```python
from build123d import *

# Parameters (mm, degrees)
F0_W      = 254
F0_H      = 409.575
F1_DEPTH  = 184.15
F2_W      = 193.675
F2_H      = 476.25
F3_DEPTH  = 95.25
F5_R      = 30.1625
F6_DEPTH  = 25.4
F7_R      = 26.9875
F8_DEPTH  = 25.4
F9_R      = 82.55
F10_DEPTH = 19.05
F11_W     = 177.8
F11_H     = 15.875
F12_DEPTH = 136.525
F14_DEPTH = 60.325
F16_DEPTH = 193.675
F17_R     = 9.525
F18_DEPTH = 38.1
F19_W     = 19.05
F19_H     = 63.5
F20_DEPTH = 12.7


with BuildPart() as f1:
    # F0 (on Top) → F1 (new body)
    with BuildSketch(Plane.XY):
        Rectangle(F0_W, F0_H)
    extrude(amount=F1_DEPTH)

    # F2 (on face) → F3 (join)
    with BuildSketch(Plane.XY.offset(184.15)):
        with Locations((30.1625, -33.3375)):
            Rectangle(F2_W, F2_H)
    extrude(amount=F3_DEPTH)

    # F5 (on face) → F6 (join)
    with BuildSketch(Plane.YZ.offset(127)):
        with Locations((141.2875, 90.4875)):
            Circle(F5_R)
    extrude(amount=F6_DEPTH)

    # F7 (on face) → F8 (cut)
    with BuildSketch(Plane.YZ.offset(152.4)):
        with Locations((141.2875, 90.4875)):
            Circle(F7_R)
    extrude(amount=-F8_DEPTH, mode=Mode.SUBTRACT)

    # F9 (on face) → F10 (join)
    with BuildSketch(Plane(origin=(-127, 0, 0), x_dir=(0, -1, 0), z_dir=(-1, 0, 0))):
        with Locations((-134.9375, 247.65)):
            Circle(F9_R)
    extrude(amount=F10_DEPTH)

    # F11 (on face) → F12 (join)
    with BuildSketch(Plane(origin=(-146.05, 0, 0), x_dir=(0, -1, 0), z_dir=(-1, 0, 0))):
        with Locations((-134.9375, 233.3625)):
            Rectangle(F11_W, F11_H)
    extrude(amount=F12_DEPTH)

    # F13 (on face) → F14 (join, through all)
    with BuildSketch(Plane(origin=(-66.675, 0, 0), x_dir=(0, -1, 0), z_dir=(-1, 0, 0))):
        with BuildLine():
            Line((-204.7875, 279.4), (-204.7875, 184.15))
            Line((-204.7875, 184.15), (15.268247, 184.15))
            ThreePointArc((15.268247, 184.15), (-74.48391, 278.617919), (-204.7875, 279.4))
        make_face()
    extrude(amount=F14_DEPTH)

    # F15 (on face) → F16 (cut, through all)
    with BuildSketch(Plane(origin=(-66.675, 0, 0), x_dir=(0, -1, 0), z_dir=(-1, 0, 0))):
        with BuildLine():
            ThreePointArc((223.8375, 279.4), (257.51346, 265.45096), (271.4625, 231.775))
            Line((271.4625, 231.775), (271.4625, 279.4))
            Line((271.4625, 279.4), (223.8375, 279.4))
        make_face()
        with BuildLine():
            ThreePointArc((271.4625, 231.775), (257.51346, 198.09904), (223.8375, 184.15))
            Line((223.8375, 184.15), (271.4625, 184.15))
            Line((271.4625, 184.15), (271.4625, 231.775))
        make_face()
    extrude(amount=-F16_DEPTH, mode=Mode.SUBTRACT)

    # F17 (on face) → F18 (join)
    with BuildSketch(Plane(origin=(0, 204.7875, 0), x_dir=(-1, 0, 0), z_dir=(0, 1, 0))):
        with Locations((136.525, 212.725)):
            Circle(F17_R)
    extrude(amount=F18_DEPTH)

    # F19 (on face) → F20 (join)
    with BuildSketch(Plane(origin=(0, 242.8875, 0), x_dir=(-1, 0, 0), z_dir=(0, 1, 0))):
        with Locations((136.525, 244.475)):
            Rectangle(F19_W, F19_H)
    extrude(amount=-F20_DEPTH)


solid = f1.part
```
Geometry: final body of the model. Coordinates: model frame, mm. A direction names the side the tool comes from. Coordinates: 2 decimals unless noted, no trailing zeros. Order: outer loops, then holes, each group sorted by start corner. A loop starts at its lowest first (then second) coordinate and runs counter-clockwise, first axis right, second up.
Item 1: Material intervals for line 1 along Z through (x, y) = (-104, -181); line 2 along Z through (x, y) = (124, 60.5); line 3 along X through (y, z) = (140.5, 20.5), sorted ascending.
Answer:
line 1: z = 0 to 184.15
line 2: z = 0 to 279.4
line 3: x = -127 to 127
Item 2: Section query C-C (y = -63.5). Output: boundary loops of the cut face in (x, z) (3 decimals).
Answer:
outline: (-127, 0) - (127, 0) - (127, 279.4) - (-66.675, 279.4) - (-66.675, 184.15) - (-127, 184.15) - close
Item 3: Access query for faces 1 (the face through (29, -7, 279.4)), 2 (the face through (139.52, 155.21, 63.73)), 3 (the face through (-213, 46.037, 233)). Directions: +Z, -Z, +X, -X, +Y, -Y. A direction counts if a zero-diameter tool reaches every point of the face in a straight line with its end or side. Return the directions, or none.
Answer:
face 1: +Z, +X, +Y, -Y
face 2: +X
face 3: +Z, -Z, -X, -Y
Item 4: Section query D-D (z = 32). Output: boundary loops of the cut face in (x, y).
Answer:
outline: (-127, -204.79) - (127, -204.79) - (127, 204.79) - (-127, 204.79) - close
Item 5: Contact query for flat-ended pins moving along their axis: P1, Ø4, axis at y = 158, z = 283, coming from the +X side (3 decimals); P2, Ø6.5, axis at y = 238, z = 233.5, coming from the +X side; P3, Ø1, axis at y = -188.5, z = 147.5, coming from the +X side. Output: stop coordinate, or through.
Answer:
P1: stops at x = -66.675
P2: stops at x = -127
P3: stops at x = 127
